Geometry check sheet. Reference: the model listing, model coordinates, mm. A direction names the side the tool comes from. Give positions to 0.01 mm unless a question says otherwise; leave off trailing zeros. One line per item, written item: value. Start each with the question number.
(1) Gauge pin test, flat ends, axial feed: pin 1 Ø5 at (y, z) = (0, 57.5) entering from +X (3 decimals); pin 2 Ø3 at (y, z) = (0.5, 61) entering from +X; pin 3 Ø10 at (y, z) = (4.5, 36.5) entering from -X. Record the tip position at first contact, or that the pin passes through.
(2) Scan lines: line 1 along Z through (x, y) = (-8, -18.5); line 2 along Y through (x, z) = (-16, 25.5); line 3 along Y through (x, z) = (23, 44). Record each from-to range of solid material in increasing order. Write a range as from..to.
(3) Tool access check on faces 1 (the face through (-14.985, 0.66, 7.049)), 2 (the face through (0, 0, 0)). Record the directions out of +Z, -Z, +X, -X, +Y, -Y that give a thin tool (end or side, any length) a straight path to the whole face; none if there is none.
from build123d import *


with BuildPart() as f1:
    # F0 (on Front) → F1 (revolve)
    with BuildSketch(Plane.XZ):
        with BuildLine():
            Line((0, 17.4324345394), (0, 0))
            Line((0, 0), (15, 0))
            Line((15, 0), (15, 13.903540875))
            ThreePointArc((15, 13.903540875), (15.5646049408, 17.2161410738), (17.1946640153, 20.1546791847))
            add(Edge.make_bspline(
                [(17.1946640153, 20.1546791847), (19.2820687523, 22.7610677336), (21.3061725207, 25.3630195661), (23.0850826912, 27.947785967)],
                knots=[0.0438155979, 0.0438155979, 0.0438155979, 0.0438155979, 0.1697178469, 0.1697178469, 0.1697178469, 0.1697178469], degree=3))
            add(Edge.make_bspline(
                [(23.0850826912, 27.947785967), (24.3132478505, 29.7323167944), (25.4245398901, 31.5086560743), (26.3591006498, 33.272608394)],
                knots=[0.1697178469, 0.1697178469, 0.1697178469, 0.1697178469, 0.2566411543, 0.2566411543, 0.2566411543, 0.2566411543], degree=3))
            ThreePointArc((26.3591006498, 33.272608394), (28.4728772846, 39.383993976), (29.1891884869, 45.8108115131))
            add(Edge.make_bspline(
                [(29.1891884869, 45.8108115131), (27.5186066734, 56.1054005015), (13.7593033367, 65.5527002508), (0, 75)],
                knots=[0.4671507953, 0.4671507953, 0.4671507953, 0.4671507953, 1, 1, 1, 1], degree=3))
            Line((0, 75), (0, 17.4324345394))
        make_face()
        with BuildLine():
            ThreePointArc((29.1891884869, 45.8108115131), (20.6398731164, 66.4506846295), (0, 75))
            add(Edge.make_bspline(
                [(29.1891884869, 45.8108115131), (27.5186066734, 56.1054005015), (13.7593033367, 65.5527002508), (0, 75)],
                knots=[0.4671507953, 0.4671507953, 0.4671507953, 0.4671507953, 1, 1, 1, 1], degree=3))
        make_face()
    revolve(axis=Axis((0, 0, 37.5), (0, 0, 1)))


solid = f1.part
Calculated:
1. pin 1: stops at x = 27.705
1. pin 2: stops at x = 25.78
1. pin 3: stops at x = -28.7
2. line 1: z = 23.93..66.92
2. line 2: y = -14.12..14.12
2. line 3: y = -17.88..17.88
3. face 1: -Z
3. face 2: -Z, +X, -X, +Y, -Y
